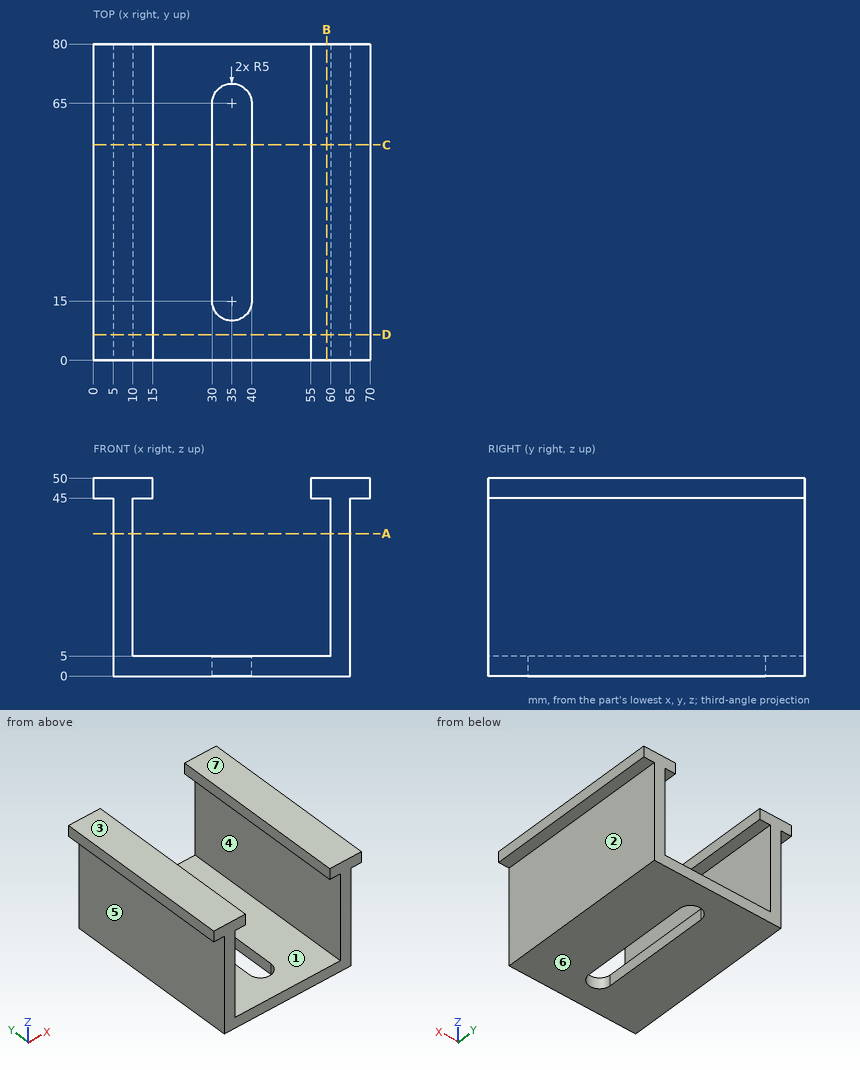
Geometry: see drawing. Coordinates: mm, zero at the bounding-box minimum. A direction names the side the tool comes from. Coordinates: 2 decimals unless noted, no trailing zeros. Write each loop counter-clockwise with the first axis right and the second up, starting at its lowest first coordinate (ties: lowest second). Pieces come first, ordered by that corner, then holes. Notation, with made-up numbers: M 74.5,-35.5 L 127.5,-35.5 A17 cw 127.5,-23.5 Z; hole C 83,68 d1. An arc over 180 degrees is marked long. Use CSV: the item, a comma, the result in double quotes. Start each with the question number.
1. Cut plane B-B on x = 59. Return the cut outline in (y, z), plus the area to 3 significant figures.
2. Cut plane C-C on y = 54.5. Return the cut outline in (x, z), plus the area to 3 significant figures.
3. Reachability of the marked faces 1, 2 and 3 from +Z, -Z, +X, -X, +Y, -Y: full face, straight path, thin tool, end or side. Return the list, or none.
4. Ray query, probe 1 along X at (y, z) = (35.5, 19); probe 2 along Z at (x, y) = (58.5, 58); probe 3 along Z at (x, y) = (41.5, 57.5). Return the intervals inside material, ascending.
5. Cut plane A-A on z = 36. Return the cut outline in (x, y).
6. Mould query, pull axis Z, two halves, no side actions, for the marked faces 4, 5, 6 and 7. Classes: pulls with the +Z half, pulls with the -Z half, needs draft (parallel to the pull), parting line crosses it, or undercut.
7. First-contact query: P1, Ø2.5, axis at x = 68.5, y = 38.5, coming from the -Z side; P2, Ø5.5, axis at y = 34, z = 3, coming from the -X side; P3, Ø22.5, axis at y = 36.5, z = 15, coming from the +X side. Flat tips, straight axial feed; report the tip coordinate or a pass-through.
8. Cut plane D-D on y = 6.5. Return the cut outline in (x, z).
Entries:
1,outline,"M 0,0 L 80,0 L 80,5 L 0,5 Z; M 0,45 L 80,45 L 80,50 L 0,50 Z"
1,area,"800 mm²"
2,outline,"M 0,45 L 5,45 L 5,0 L 30,0 L 30,5 L 10,5 L 10,45 L 15,45 L 15,50 L 0,50 Z; M 40,0 L 65,0 L 65,45 L 70,45 L 70,50 L 55,50 L 55,45 L 60,45 L 60,5 L 40,5 Z"
2,area,"800 mm²"
3,face 1,"+Y, -Y"
3,face 2,"-Z, +X, +Y, -Y"
3,face 3,"+Z, +X, -X, +Y, -Y"
4,probe 1,"5 to 10, 60 to 65"
4,probe 2,"0 to 5, 45 to 50"
4,probe 3,"0 to 5"
5,outline,"M 5,0 L 10,0 L 10,80 L 5,80 Z; M 60,0 L 65,0 L 65,80 L 60,80 Z"
6,face 4,"undercut"
6,face 5,"needs draft"
6,face 6,"pulls with the -Z half"
6,face 7,"pulls with the +Z half"
7,P1,"z = 45"
7,P2,"x = 5"
7,P3,"x = 65"
8,outline,"M 0,45 L 5,45 L 5,0 L 65,0 L 65,45 L 70,45 L 70,50 L 55,50 L 55,45 L 60,45 L 60,5 L 10,5 L 10,45 L 15,45 L 15,50 L 0,50 Z"
